The listing builds one solid part. Answer for the finished solid, in the listing's coordinates (mm). A direction names the side the tool comes from. Round coordinates to 2 decimals unless told otherwise and drop trailing zeros. Write each loop counter-clockwise with the first axis right and the second up, starting at its lowest first coordinate (ties: lowest second). Pieces come first, ordered by that corner, then holes.
from build123d import *

# Parameters (mm, degrees)
SKETCH_1_R      = 11.5
SKETCH_1_R_2    = 1.5
SKETCH_1_W      = 36
SKETCH_1_H      = 15
EXTRUDE_1_DEPTH = 5


with BuildPart() as part:
    # 草图1 → 凸台-拉伸1 (new body)
    with BuildSketch(Plane.XY):
        Polygon((-2.5, 100), (15, 100), (15, 105), (45, 105), (45, 100), (55, 100), (55, 0), (45, 0), (45, -5), (15, -5), (15, 0), (-2.5, 0), (-2.5, 15), (-7.5, 15), (-7.5, 45), (-2.5, 45), align=None)
        with Locations((30, 30)):
            Circle(SKETCH_1_R, mode=Mode.SUBTRACT)
        with Locations((14.5, 45.5)):
            Circle(SKETCH_1_R_2, mode=Mode.SUBTRACT)
        with Locations((45.5, 45.5)):
            Circle(SKETCH_1_R_2, mode=Mode.SUBTRACT)
        with Locations((45.5, 14.5)):
            Circle(SKETCH_1_R_2, mode=Mode.SUBTRACT)
        with Locations((14.5, 14.5)):
            Circle(SKETCH_1_R_2, mode=Mode.SUBTRACT)
        with Locations((26.25, 77.5)):
            Rectangle(SKETCH_1_W, SKETCH_1_H, mode=Mode.SUBTRACT)
    extrude(amount=EXTRUDE_1_DEPTH)


solid = part.part
1. A tool of negligible diameter and unlimited length cuts with its end or side. For faces 1 (the face through (45, -2, 2)), 2 (the face through (50, 100, 2)), 3 (the face through (6, 100, 2)), 4 (the face through (15, -3, 2)), from which of +Z, -Z, +X, -X, +Y, -Y can it reach the whole face along a straight path? Write none if from no direction.
Geometry says:
face 1: +Z, -Z, +X, -Y
face 2: +Z, -Z, +X, +Y
face 3: +Z, -Z, -X, +Y
face 4: +Z, -Z, -X, -Y
2. Straight lines are drawn through the part: line 1 along Y through (x, z) = (45.5, 1.9); line 2 along X through (y, z) = (73, 2.85); line 3 along Y through (x, z) = (14.5, 2.05). For each, find the intervals that lie inside material, in ascending order.
Geometry says:
line 1: y = 0 to 13, 16 to 44, 47 to 100
line 2: x = -2.5 to 8.25, 44.25 to 55
line 3: y = 0 to 13, 16 to 44, 47 to 70, 85 to 100
3. Section C-C on z = 0.75 is taken. Determine the outline of the cut face in (x, y), plus the area to 3 significant figures.
Geometry says:
outline: (-7.5, 15) - (-2.5, 15) - (-2.5, 0) - (15, 0) - (15, -5) - (45, -5) - (45, 0) - (55, 0) - (55, 100) - (45, 100) - (45, 105) - (15, 105) - (15, 100) - (-2.5, 100) - (-2.5, 45) - (-7.5, 45) - close; hole (8.25, 70) - (44.25, 70) - (44.25, 85) - (8.25, 85) - close; hole circle Ø3 at (14.5, 14.5); hole circle Ø3 at (14.5, 45.5); hole circle Ø23 at (30, 30); hole circle Ø3 at (45.5, 14.5); hole circle Ø3 at (45.5, 45.5)
area: 5,220 mm2
4. Section A-A on x = 30 is taken. Determine the outline of the cut face in (y, z), plus the area to 3 significant figures.
Geometry says:
outline: (-5, 0) - (18.5, 0) - (18.5, 5) - (-5, 5) - close; (41.5, 0) - (70, 0) - (70, 5) - (41.5, 5) - close; (85, 0) - (105, 0) - (105, 5) - (85, 5) - close
area: 360 mm2
5. Section D-D on x = 0.5 is taken. Determine the outline of the cut face in (y, z), plus the area to 3 significant figures.
Geometry says:
outline: (0, 0) - (100, 0) - (100, 5) - (0, 5) - close
area: 500 mm2
6. For a pull along X with two mould halves and no side action, classify faces 5 (the face through (55, 51, 2)), 6 (the face through (-5, 15, 2)), 7 (the face through (14.175, 44.036, 2.465)) as released by +X, released by -X, zero draft, split by the parting line, or undercut.
Geometry says:
face 5: released by +X
face 6: zero draft
face 7: undercut
7. Given pin 1 (1.5 mm diameter, centred on x = -4, z = 1.5, fed in from -Y); pin 2 (1.5 mm diameter, centred on y = 81, z = 2.5, fed in from -X); pin 3 (2.5 mm diameter, centred on y = -3, z = 1.5, fed in from -X); pin 4 (3.5 mm diameter, centred on x = 14.5, y = 14.5, fed in from +Z), each flat-ended and moving along its own axis, determine where each tip first touches the part or whether it passes through.
Geometry says:
pin 1: stops at y = 15
pin 2: stops at x = -2.5
pin 3: stops at x = 15
pin 4: stops at z = 5
8. Section B-B on y = 30 is taken. Determine the outline of the cut face in (x, z), plus the area to 4 significant figures.
Geometry says:
outline: (-7.5, 0) - (18.5, 0) - (18.5, 5) - (-7.5, 5) - close; (41.5, 0) - (55, 0) - (55, 5) - (41.5, 5) - close
area: 197.5 mm2
